```python
from build123d import *

# Parameters (mm, degrees)
SKETCH1_R           = 12.5
BOSS_EXTRUDE1_DEPTH = 1.6
SKETCH2_R           = 11
BOSS_EXTRUDE2_DEPTH = 16
SKETCH3_R           = 12.5
BOSS_EXTRUDE3_DEPTH = 1.6
SKETCH4_R           = 11
BOSS_EXTRUDE4_DEPTH = 7
SKETCH5_R           = 4
CUT_EXTRUDE1_DEPTH  = 27.2


with BuildPart() as part:
    # Sketch1 → Boss-Extrude1 (new body)
    with BuildSketch(Plane(origin=(0, 0, 0), x_dir=(1, 0, 0), z_dir=(0, 1, 0))):
        Circle(SKETCH1_R)
    extrude(amount=BOSS_EXTRUDE1_DEPTH)

    # Sketch2 → Boss-Extrude2 (add)
    with BuildSketch(Plane(origin=(0, 1.6, 0), x_dir=(1, 0, 0), z_dir=(0, 1, 0))):
        Circle(SKETCH2_R)
    extrude(amount=BOSS_EXTRUDE2_DEPTH)

    # Sketch3 → Boss-Extrude3 (add)
    with BuildSketch(Plane(origin=(0, 17.6, 0), x_dir=(1, 0, 0), z_dir=(0, 1, 0))):
        Circle(SKETCH3_R)
    extrude(amount=BOSS_EXTRUDE3_DEPTH)

    # Sketch4 → Boss-Extrude4 (add)
    with BuildSketch(Plane(origin=(0, 19.2, 0), x_dir=(1, 0, 0), z_dir=(0, 1, 0))):
        Circle(SKETCH4_R)
    extrude(amount=BOSS_EXTRUDE4_DEPTH)

    # Sketch5 → Cut-Extrude1 (cut, through all)
    with BuildSketch(Plane.XZ):
        Circle(SKETCH5_R)
    extrude(amount=-CUT_EXTRUDE1_DEPTH, mode=Mode.SUBTRACT)


solid = part.part
```
Design review of the part built by this model. Coordinates are the model's own, in mm. A direction names the side the tool comes from. Coordinates: 2 decimals unless noted, no trailing zeros. Loops run counter-clockwise (first coordinate to the right, second up) from the corner with the lowest first, then second, coordinate; pieces in that order, holes last. Notation, with made-up numbers: M 81,-35 L 117,-35 A21 ccw 117,-2 Z; hole C 54.25,31.25 d8. An arc over 180 degrees is marked long. One line per question, with ' | ' between items.
(1) Wall thickness on probe 1 along Z at (x, y) = (0, 12.5); probe 2 along Y at (x, z) = (-9.75, 6); probe 3 along Z at (x, y) = (0, 17.75): over which ranges is each line inside the solid? List them lowest first.
Filled in:
probe 1: z = -11 to -4, 4 to 11 | probe 2: y = 0 to 1.6, 17.6 to 19.2 | probe 3: z = -12.5 to -4, 4 to 12.5
(2) Draft analysis for pull direction Y (two halves, no side actions). For faces 1 (the face through (0, 26.2, 5)), 2 (the face through (5, 1.6, 10)), 3 (the face through (-2.38, 22.65, 10.74)), 4 (the face through (-3, 0, -3)), state which applies: released by +Y, released by -Y, zero draft, split by the parting line, or undercut.
Filled in:
face 1: released by +Y | face 2: undercut | face 3: zero draft | face 4: released by -Y
(3) For pin 1 Ø3 at (x, y) = (-9, 22) entering from +Z; pin 2 Ø5 at (x, z) = (0, 0) entering from -Y; pin 3 Ø3 at (y, z) = (13.5, 6) entering from +X; pin 4 Ø10 at (y, z) = (12, 1) entering from +X, all flat-tipped, find the tip position at first contact; note any pin that passes through.
Filled in:
pin 1: stops at z = 8.05 | pin 2: passes through | pin 3: stops at x = 10.04 | pin 4: stops at x = 11
(4) We need section B-B (z = 0). Give the boundary of the cut face in (x, y).
Filled in:
outline: M -12.5,0 L -4,0 L -4,26.2 L -11,26.2 L -11,19.2 L -12.5,19.2 L -12.5,17.6 L -11,17.6 L -11,1.6 L -12.5,1.6 Z; M 4,0 L 12.5,0 L 12.5,1.6 L 11,1.6 L 11,17.6 L 12.5,17.6 L 12.5,19.2 L 11,19.2 L 11,26.2 L 4,26.2 Z
(5) Machinability: for faces 5 (the face through (5, 17.6, 10)), 6 (the face through (5, 19.2, 10)), 7 (the face through (11.923, 18.389, -3.755)), which of the approach directions +Z, -Z, +X, -X, +Y, -Y give a long, thin tool a straight path to every point of the face, cutting with its end or side? Answer none if there is none.
Filled in:
face 5: none | face 6: +Y | face 7: +Y, -Y
(6) We need section D-D (z = -6). Give the boundary of the cut face in (x, y).
Filled in:
outline: M -10.97,0 L 10.97,0 L 10.97,1.6 L 9.22,1.6 L 9.22,17.6 L 10.97,17.6 L 10.97,19.2 L 9.22,19.2 L 9.22,26.2 L -9.22,26.2 L -9.22,19.2 L -10.97,19.2 L -10.97,17.6 L -9.22,17.6 L -9.22,1.6 L -10.97,1.6 Z
(7) We need section C-C (y = 5). Give the boundary of the cut face in (x, z), and give its area (3 significant figures).
Filled in:
outline: C 0,0 d22; hole C 0,0 d8 | area: 330 mm^2
(8) We need section A-A (x = 0). Give the boundary of the cut face in (y, z), and give its area (3 significant figures).
Filled in:
outline: M 0,-12.5 L 1.6,-12.5 L 1.6,-11 L 17.6,-11 L 17.6,-12.5 L 19.2,-12.5 L 19.2,-11 L 26.2,-11 L 26.2,-4 L 0,-4 Z; M 0,4 L 26.2,4 L 26.2,11 L 19.2,11 L 19.2,12.5 L 17.6,12.5 L 17.6,11 L 1.6,11 L 1.6,12.5 L 0,12.5 Z | area: 376 mm^2
